Part print with two shaded views. Sizes in mm from the minimum x, y, z corner. Give positions to 0.01 mm unless a question says otherwise; leave off trailing zeros. Write each loop counter-clockwise with the first axis right and the second up, starting at its lowest first coordinate (ties: lowest second). Pieces come first, ordered by that corner, then holes. Notation, with made-up numbers: M 45.5,63 L 96.5,63 A18 ccw 96.5,76 Z; hole C 76,30.25 d8. An arc over 180 degrees is marked long. Return JSON: item names as keys, results as strings. Group by question number.
Q1. Band-saw the part on A-A, the plane x = 21. Give the cut face in (y, z), then the cut area to 3 significant figures.
Q2. Band-saw the part on D-D, the plane x = 5.5. Give the cut face in (y, z).
Q3. Band-saw the part on B-B, the plane z = 21. Give the cut face in (x, y), then the cut area to 3 significant figures.
Q4. Wall check: probe 1 along Z at (x, y) = (36.5, 2.25); probe 2 along X at (y, z) = (1.55, 37). Give the ranges that are in metal, low to high.
Q5. Flat gauge pins, fed straight in: pin 1 Ø4.5 at (x, z) = (36.5, 5.5) entering from +Y; pin 2 Ø3 at (x, z) = (36.5, 36.5) entering from -Y. Where does each tip first touch, or does it go through?
Q6. Band-saw the part on C-C, the plane z = 5.5. Give the cut face in (x, y).
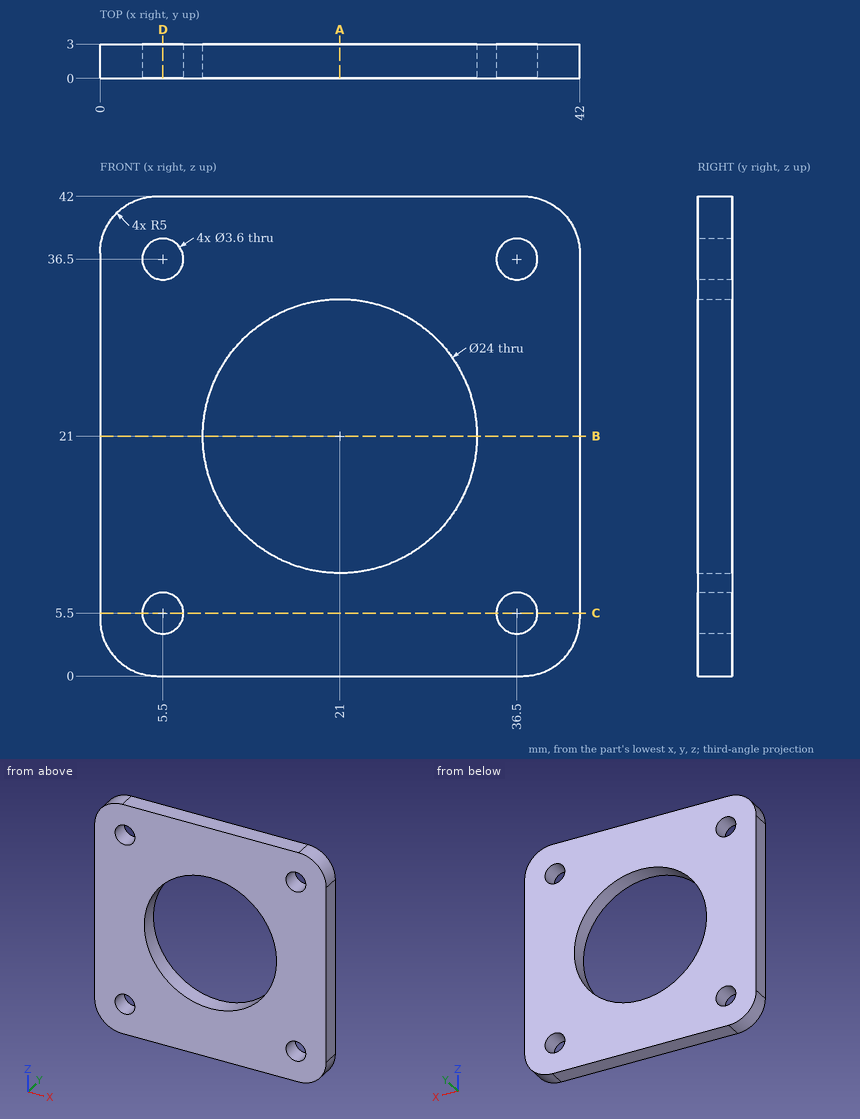
From the geometry:
{
 "1": {"outline": "M 0,0 L 3,0 L 3,9 L 0,9 Z; M 0,33 L 3,33 L 3,42 L 0,42 Z", "area": "54.0 mm^2"},
 "2": {"outline": "M 0,0 L 3,0 L 3,3.7 L 0,3.7 Z; M 0,7.3 L 3,7.3 L 3,34.7 L 0,34.7 Z; M 0,38.3 L 3,38.3 L 3,42 L 0,42 Z"},
 "3": {"outline": "M 0,0 L 9,0 L 9,3 L 0,3 Z; M 33,0 L 42,0 L 42,3 L 33,3 Z", "area": "54.0 mm^2"},
 "4": {"probe 1": "z = 0 to 3.7, 7.3 to 34.7, 38.3 to 42", "probe 2": "x = 0 to 3.77, 7.23 to 34.77, 38.23 to 42"},
 "5": {"pin 1": "stops at y = 3", "pin 2": "passes through"},
 "6": {"outline": "M 0,0 L 3.7,0 L 3.7,3 L 0,3 Z; M 7.3,0 L 34.7,0 L 34.7,3 L 7.3,3 Z; M 38.3,0 L 42,0 L 42,3 L 38.3,3 Z"}
}
